Design review of the part built by this model. Coordinates are the model's own, in mm. A direction names the side the tool comes from. Coordinates: 2 decimals unless noted, no trailing zeros. Write each loop counter-clockwise with the first axis right and the second up, starting at its lowest first coordinate (ties: lowest second). Pieces come first, ordered by that corner, then holes. Notation, with made-up numbers: (16.25, 61.25) - (25.25, 61.25) arc R29 cw to (25.25, 98.25) - close; hole circle Ø8 at (33, -26). An arc over 180 degrees is marked (long way). One line per item, written item: value.
Autodesk Inventor part; units mm, degrees
ref_plane "YZ Plane" through (0, 0, 0) normal (1, 0, 0) x (0, 1, 0)
ref_plane "XZ Plane" through (0, 0, 0) normal (0, 1, 0) x (-1, 0, 0)
ref_plane "XY Plane" through (0, 0, 0) normal (0, 0, 1) x (1, 0, 0)
sketch "Sketch1" plane through (0, 0, 0) normal (0, 0, 1) x (1, 0, 0)
  circle A0 centre (0, 0) radius 9.525 construction
  circle A1 centre (0, 0) radius 2.54 construction
  line L0 (-15.875, 0.5) -> (-2.4903, 0.5)
  line L1 (2.4903, 0.5) -> (15.875, 0.5)
  line L2 (15.875, 0.5) -> (15.875, 5.5)
  line L3 (15.875, 5.5) -> (7.7766, 5.5)
  line L4 (-15.875, 0.5) -> (-15.875, 5.5)
  line L5 (-15.875, 5.5) -> (-7.7766, 5.5)
  arc A2 (2.4903, 0.5) -> (-2.4903, 0.5) centre (0, 0) ccw
  arc A3 (7.7766, 5.5) -> (-7.7766, 5.5) centre (0, 0) ccw
  dimension "d0" = 5.08
  dimension "d2" = 19.05
  dimension "d3" = 0.5
  dimension "d4" = 5
  dimension "d5" = 15.875
extrude "Extrusion1" add sketch "Sketch1" along normal blind 12.7
sketch "Sketch3" plane through (7.7766, 5.5, 0) normal (0, 1, 0) x (1, 0, 0)
  line L0 (8.0984, 0) -> (8.0984, -12.7)
  line L1 (-15.5532, 0) -> (0, 0)
  line L2 (-15.5532, 0) -> (-23.6516, 0)
  line L3 (-23.6516, 0) -> (-23.6516, -12.7)
  line L4 (-15.5532, -12.7) -> (-23.6516, -12.7)
  line L5 (-15.5532, 0) -> (-15.5532, -12.7)
  circle A0 centre (-19.6829, -6.35) radius 1.6
  circle A1 centre (4.1296, -6.35) radius 1.6
  point P0 (-7.7766, 0)
  point P1 (-23.6516, -6.35)
  point P2 (8.0984, -6.35)
  point P3 (-7.7766, 0)
  dimension "d13" = 3.2
  dimension "d15" = 11.9062
  dimension "d16" = 11.9062
extrude "Extrusion3" cut sketch "Sketch3" against normal through all contours A0 | A1
sketch "Sketch2" plane through (0, 0, 0) normal (0, 0, -1) x (-1, 0, 0)
  line L0 (15.875, 0.5) -> (2.4903, 0.5)
  line L1 (-2.4903, 0.5) -> (-15.875, 0.5)
  arc A0 (2.4903, 0.5) -> (-2.4903, 0.5) centre (0, 0) ccw
  arc A1 (7.9217, 0.5) -> (-7.9217, 0.5) centre (0, 0) ccw
  dimension "d8" = 7.9375
extrude "Extrusion2" add sketch "Sketch2" along normal blind 1.5875
sketch "Sketch6" plane through (7.7766, 5.5, 0) normal (0, 1, 0) x (1, 0, 0)
  circle A0 centre (4.1296, -6.35) radius 1.6
  line L0 (8.0984, 0) -> (0, 0)
  line L1 (8.0984, -12.7) -> (0, -12.7)
  line L2 (8.0984, 0) -> (8.0984, -12.7)
  line L3 (2.5131, -3.55) -> (5.7462, -3.55)
  line L4 (5.7462, -3.55) -> (7.3628, -6.35)
  line L5 (7.3628, -6.35) -> (5.7462, -9.15)
  line L6 (5.7462, -9.15) -> (2.5131, -9.15)
  line L7 (2.5131, -9.15) -> (0.8965, -6.35)
  line L8 (0.8965, -6.35) -> (2.5131, -3.55)
  line L9 (0, 0) -> (-8.0984, 0)
  line L10 (-8.0984, 0) -> (-8.0984, -12.7)
  line L11 (-8.0984, -12.7) -> (0, -12.7)
  line L12 (0, -12.7) -> (0, 0)
  point P0 (-7.7766, 0)
  dimension "d30" = 5.6
extrude "Extrusion5" add sketch "Sketch6" along normal blind 3 contours L2 L1 L12 L0 | L12 L11 L10 L9
properties part number "THREAD CLAMP"
1. Consider section B-B, the plane z = 5.5. Write out the cut boundary in (x, y) (3 decimals).
Answer block:
outline: (-15.875, 0.5) - (-13.262, 0.5) - (-13.262, 5.5) - (-15.875, 5.5) - close; (-10.551, 0.5) - (-2.49, 0.5) arc R2.54 cw to (2.49, 0.5) - (10.551, 0.5) - (10.551, 5.5) - (9.164, 5.5) - (9.164, 8.5) - (4.298, 8.5) arc R9.525 ccw to (-7.777, 5.5) - (-10.551, 5.5) - close; (13.262, 0.5) - (15.875, 0.5) - (15.875, 8.5) - (14.649, 8.5) - (14.649, 5.5) - (13.262, 5.5) - close
2. Insertion check: pin 1 Ø2.5 at (x, y) = (11.5, 7.5) entering from -Z; pin 2 Ø6 at (x, z) = (12, 7.5) entering from +Y; pin 3 Ø5 at (x, z) = (11.91, 6.35) entering from +Y. Each pin has a flat end and moves straight along its axis. Give the tip position at first contact, or say it passes through.
Answer block:
pin 1: stops at z = 0
pin 2: stops at y = 8.5
pin 3: stops at y = 5.5
3. Consider section A-A, the plane y = 2.25. Give the number of separate pieces and of enclosed holes in the cut face, then the cut area to 3 significant figures.
Answer block:
separate pieces: 2
enclosed holes: 2
area: 378 mm^2
4. Mouldability with a two-part tool opening along Z and no side actions: class faces 5 (the face through (9.493, 6.979, 7.77)), 6 (the face through (0, 4, 12.7)), 7 (the face through (0, 4, -1.588)), 8 (the face through (0.05, 2.54, 5.66)) as released by +Z, released by -Z, zero draft, split by the parting line, or undercut.
Answer block:
face 5: undercut
face 6: released by +Z
face 7: released by -Z
face 8: zero draft
5. Consider section C-C, the plane x = -11. Write out the cut boundary in (y, z), then the cut area to 3 significant figures.
Answer block:
outline: (0.5, 0) - (5.5, 0) - (5.5, 5.03) - (0.5, 5.03) - close; (0.5, 7.67) - (5.5, 7.67) - (5.5, 12.7) - (0.5, 12.7) - close
area: 50.3 mm^2
6. Consider section D-D, the plane z = 1.75. Write out the cut boundary in (x, y) (3 decimals).
Answer block:
outline: (-15.875, 0.5) - (-2.49, 0.5) arc R2.54 cw to (2.49, 0.5) - (15.875, 0.5) - (15.875, 8.5) - (4.298, 8.5) arc R9.525 ccw to (-7.777, 5.5) - (-15.875, 5.5) - close
7. Wall thickness on line 1 along X through (y, z) = (2.95, 6.35) (3 decimals); line 2 along X through (y, z) = (2, 6.35) (3 decimals); line 3 along Y through (x, z) = (5, 9.5): over which ranges is each line inside the solid? List them lowest first.
Answer block:
line 1: x = -15.875 to -13.506, -10.306 to 10.306, 13.506 to 15.875
line 2: x = -15.875 to -13.506, -10.306 to -1.566, 1.566 to 10.306, 13.506 to 15.875
line 3: y = 0.5 to 8.5
8. For faces 1 (the face through (-11, 5.5, 4.8)), 2 (the face through (14.342, 6.979, 7.73)), 3 (the face through (0.168, 7.936, -0.783)), 4 (the face through (9, 8.5, 5)), list the 3-axis set-ups (+Z, -Z, +X, -X, +Y, -Y) from which the entire face can be reached by the end or side of a thin tool; tool diameter is ignored.
Answer block:
face 1: +Z, -Z, -X, +Y
face 2: +Y
face 3: -Z, +Y
face 4: +Z, -Z, +X, +Y
